Autodesk Inventor part; units mm, degrees
ref_plane "YZ Plane" through (0, 0, 0) normal (1, 0, 0) x (0, 1, 0)
ref_plane "XZ Plane" through (0, 0, 0) normal (0, 1, 0) x (-1, 0, 0)
ref_plane "XY Plane" through (0, 0, 0) normal (0, 0, 1) x (1, 0, 0)
sketch "Sketch1" plane through (0, 0, 0) normal (0, 0, 1) x (1, 0, 0)
  line L0 (-35.5, 13.25) -> (35.5, 13.25)
  line L1 (35.5, 13.25) -> (35.5, -13.25)
  line L2 (35.5, -13.25) -> (-35.5, -13.25)
  line L3 (-35.5, -13.25) -> (-35.5, 13.25)
  point P0 (0, 0)
  dimension "d0" = 26.5
  dimension "d1" = 71
  dimension "d2" = 35.5
  dimension "d3" = 13.25
extrude "Extrusion1" add sketch "Sketch1" along normal blind 1.2
fillet "Fillet1" radius 3.25 4 edges at (-35.5, 13.25, 0.6) (-35.5, -13.25, 0.6) (35.5, -13.25, 0.6) (35.5, 13.25, 0.6)
sketch "Sketch2" plane through (0, 0, 1.2) normal (0, 0, 1) x (1, 0, 0)
  line L0 (32.25, 13.25) -> (-32.25, 13.25)
  line L1 (-35.5, 10) -> (-35.5, -10)
  line L2 (-32.25, -13.25) -> (32.25, -13.25)
  line L3 (35.5, -10) -> (35.5, 10)
  point P0 (0, 0)
  point P1 (-32.5, 10.25)
  point P2 (32.5, 10.25)
  point P3 (32.5, -10.25)
  point P4 (-32.5, -10.25)
  dimension "d7" = 3
  dimension "d8" = 3
  dimension "d9" = 3
  dimension "d10" = 3
  dimension "d11" = 3
  dimension "d12" = 3
  dimension "d13" = 3
  dimension "d14" = 3
hole "Hole1" at (-32.5, 10.25, 1.2) at (32.5, 10.25, 1.2) at (32.5, -10.25, 1.2) at (-32.5, -10.25, 1.2) direction (0, 0, -1) diameter 2.5 depth 4 tip angle 118 countersink diameter 4 countersink angle 90
sketch "Sketch3" plane through (0, 0, 1.2) normal (0, 0, 1) x (1, 0, 0)
  line L0 (-27.3, -2.85) -> (-18.3, -2.85)
  line L1 (-18.3, -2.85) -> (-18.3, -7.05)
  line L2 (-18.3, -7.05) -> (-27.3, -7.05)
  line L3 (-27.3, -7.05) -> (-27.3, -2.85)
  line L4 (-35.5, 10) -> (-35.5, -10)
  line L5 (-32.25, -13.25) -> (32.25, -13.25)
  point P0 (0, 0)
  dimension "d22" = 8.2
  dimension "d23" = 17.2
  dimension "d24" = 6.2
  dimension "d25" = 10.4
  dimension "d29" = 9
  dimension "d30" = 4.2
extrude "Extrusion2" cut sketch "Sketch3" against normal blind 1.2
fillet "Fillet2" radius 1 4 edges at (-27.3, -2.85, 0.6) (-27.3, -7.05, 0.6) (-18.3, -2.85, 0.6) (-18.3, -7.05, 0.6)
sketch "Sketch4" plane through (0, 0, 0) normal (0, 0, -1) x (-1, 0, 0)
  line L0 (-29.5, 8.25) -> (29.5, 8.25)
  line L1 (29.5, 8.25) -> (29.5, 6.25)
  line L2 (29.5, 6.25) -> (-29.5, 6.25)
  line L3 (-29.5, 6.25) -> (-29.5, 8.25)
  line L4 (-35.5, -10) -> (-35.5, 10)
  line L5 (35.5, 10) -> (35.5, -10)
  line L6 (-32.25, 13.25) -> (32.25, 13.25)
  point P0 (0, 0)
  dimension "d31" = 6
  dimension "d32" = 6
  dimension "d33" = 2
  dimension "d34" = 5
extrude "Extrusion3" add sketch "Sketch4" along normal blind 3
chamfer "Chamfer1" distance 3 angle 45 2 edges at (29.5, 7.25, -3) (-29.5, 7.25, -3)
properties part number "cover"
Model file for the job. Use its own axes, mm. A direction names the side the tool comes from. Give positions to 0.01 mm unless a question says otherwise; leave off trailing zeros. Loops run counter-clockwise (first coordinate to the right, second up) from the corner with the lowest first, then second, coordinate; pieces in that order, holes last.
1) Tool access for faces 4 (the flat face through (-23, -7.05, 1)), 5 (the flat face through (0, 0, 1.2)): list every direction of +Z, -Z, +X, -X, +Y, -Y with a clear straight run to the whole face (end or side of a thin tool).
2) Saw through at B-B (y = 0.25). Write the cut outline in (x, z), plus the area to 3 significant figures.
3) Flat gauge pins, fed straight in: pin 1 Ø4 at (x, y) = (32.5, -10.25) entering from -Z; pin 2 Ø1 at (x, z) = (-26, -2) entering from +Y; pin 3 Ø2 at (x, y) = (-32.5, -10.25) entering from -Z; pin 4 Ø1.5 at (x, z) = (-14.5, -1.5) entering from -Y. Where does each tip first touch, or does it go through?
4) Saw through at A-A (x = 7). Write the cut outline in (y, z), plus the area to 3 significant figures.
5) Saw through at C-C (z = -1). Write the cut outline in (x, y).
6) Wall check: line 1 (X direction, y = 10.25, z = 0.2); line 2 (Y direction, x = 32.5, z = 0.35); line 3 (X direction, y = -5.5, z = 1). Give the ranges that are in metal, low to high.
7) Pull direction X, two halves, no side cores. Call faces 1 (the cylindrical face through (34.523, -12.323, 0.608)), 2 (the flat face through (-23, -2.85, 1)), 3 (the flat face through (0, 13.25, 1)): +X half, -X half, draft (parallel to the pull), parting line (faces both ways), or undercut.
Answer block:
1. face 4: +Z, -Z
1. face 5: +Z, +X, -X, +Y, -Y
2. outline: (-35.5, 0) - (35.5, 0) - (35.5, 1.2) - (-35.5, 1.2) - close
2. area: 85.2 mm2
3. pin 1: stops at z = 0
3. pin 2: stops at y = 8.25
3. pin 3: passes through
3. pin 4: stops at y = 6.25
4. outline: (-13.25, 0) - (6.25, 0) - (6.25, -3) - (8.25, -3) - (8.25, 0) - (13.25, 0) - (13.25, 1.2) - (-13.25, 1.2) - close
4. area: 37.8 mm2
5. outline: (-28.5, 6.25) - (28.5, 6.25) - (28.5, 8.25) - (-28.5, 8.25) - close
6. line 1: x = -35.49 to -33.75, -31.25 to 31.25, 33.75 to 35.49
6. line 2: y = -13.24 to -11.5, -9 to 9, 11.5 to 13.24
6. line 3: x = -35.5 to -27.3, -18.3 to 35.5
7. face 1: +X half
7. face 2: undercut
7. face 3: draft
